```python
from build123d import *

# Parameters (mm, degrees)
SKETCH009_R     = 5.75
PAD005_DEPTH    = 2.2
POCKET_DEPTH    = 1.4
CHAMFER001_SIZE = 0.7
SKETCH011_R     = 2.45
PAD006_DEPTH    = 40
SKETCH012_R     = 2.8
PAD007_DEPTH    = 57


with BuildPart() as part:
    # Sketch009 → Pad005 (new body)
    with BuildSketch(Plane.XY):
        Circle(SKETCH009_R)
    extrude(amount=PAD005_DEPTH)

    # Sketch010 (on Face3 of Pad005) → Pocket (cut)
    with BuildSketch(Plane.XY.offset(2.2)):
        Polygon((2.886751, 0), (1.443376, 2.5), (-1.443376, 2.5), (-2.886751, 0), (-1.443376, -2.5), (1.443376, -2.5), align=None)
    extrude(amount=-POCKET_DEPTH, mode=Mode.SUBTRACT)

    # Chamfer001
    chamfer001_edges = [part.edges().sort_by_distance(p)[0] for p in [
        (-5.75, 0, 2.2),
    ]]
    chamfer(chamfer001_edges, length=CHAMFER001_SIZE)

    # Sketch011 (on Face3 of Chamfer001) → Pad006 (join)
    with BuildSketch(Plane(origin=(0, 0, 0), x_dir=(1, 0, 0), z_dir=(0, 0, -1))):
        Circle(SKETCH011_R)
    extrude(amount=PAD006_DEPTH)

    # Sketch012 (on Face12 of Pad006) → Pad007 (join)
    with BuildSketch(Plane(origin=(0, 0, -40), x_dir=(1, 0, 0), z_dir=(0, 0, -1))):
        Circle(SKETCH012_R)
    extrude(amount=PAD007_DEPTH)


solid = part.part
```
Read the model definition and answer for the solid it produces. Units are mm, in the model's axes. A direction names the side the tool comes from. Give positions to 0.01 mm unless a question says otherwise; leave off trailing zeros. Write each loop counter-clockwise with the first axis right and the second up, starting at its lowest first coordinate (ties: lowest second). Pieces come first, ordered by that corner, then holes. Notation, with made-up numbers: (6.25, 75.5) - (41.25, 75.5) arc R12 ccw to (41.25, 92.5) - close; hole circle Ø9 at (-39, 2). An arc over 180 degrees is marked (long way). Write item = value, one per line. Start each with the question number.
Item 1: A tool of negligible diameter and unlimited length cuts with its end or side. For faces 4 (the cylindrical face through (-2.8, -0.1, -68.1)), 5 (the flat face through (0, 0, -97)), 6 (the cylindrical face through (-0.5, 2.4, -19.7)), from which of +Z, -Z, +X, -X, +Y, -Y can it reach the whole face along a straight path? Write none if from no direction.
Item 2: Find section B-B (z = -20.5). Give the vertices of the cut face in (x, y), then the cut area to 3 significant figures.
Item 3: Each of these flat-tipped pins is pushed along its axis until it touches: P1, Ø2, axis at x = -3, z = -29.5, coming from the +Y side; P2, Ø2, axis at y = -0.5, z = -86, coming from the -X side; P3, Ø0.7, axis at x = -0.5, z = 1.5, coming from the -Y side. Where does it stop, or does it pass through?
Item 4: Find the intervals of material crossed by probe 1 along Z at (x, y) = (4.5, 1); probe 2 along X at (y, z) = (0.25, -43); probe 3 along Z at (x, y) = (-0.5, -0.75), in increasing order. Write a range as [from, to].
Item 5: The mould has two halves that part along X. Classify faces 1 (the cylindrical face through (-0.75, 5.7, 0.74)), 2 (the flat face through (0, 0, 0.8)), 3 (the flat face through (2.5, -1.2, 0)): +X half, -X half, draft (parallel to the pull), parting line (faces both ways), or undercut.
Item 6: Find section A-A (x = 0). Give the vertices of the cut face in (y, z), then the cut area to 3 significant figures.
Item 7: Find section C-C (z = -78). Give the vertices of the cut face in (x, y), then the cut area to 3 significant figures.
Response:
q1.face_4 = -Z
q1.face_5 = -Z, +X, -X, +Y, -Y
q1.face_6 = none
q2.outline = circle Ø4.9 at (0, 0)
q2.area = 18.9 mm²
q3.P1 = 1.42
q3.P2 = -2.8
q3.P3 = -5.75
q4.probe_1 = [0, 2.2]
q4.probe_2 = [-2.79, 2.79]
q4.probe_3 = [-97, 0.8]
q5.face_1 = parting line
q5.face_2 = undercut
q5.face_3 = draft
q6.outline = (-5.75, 0) - (-2.45, 0) - (-2.45, -40) - (-2.8, -40) - (-2.8, -97) - (2.8, -97) - (2.8, -40) - (2.45, -40) - (2.45, 0) - (5.75, 0) - (5.75, 1.5) - (5.05, 2.2) - (2.5, 2.2) - (2.5, 0.8) - (-2.5, 0.8) - (-2.5, 2.2) - (-5.05, 2.2) - (-5.75, 1.5) - close
q6.area = 533 mm²
q7.outline = circle Ø5.6 at (0, 0)
q7.area = 24.6 mm²
